```python
from build123d import *

# Parameters (mm, degrees)
SKETCH_W        = 70
SKETCH_H        = 70
PAD_DEPTH       = 15
SKETCH001_R     = 26
POCKET_DEPTH    = 11
SKETCH002_R     = 3
SKETCH002_R_2   = 21
POCKET001_DEPTH = 15.001


with BuildPart() as part:
    # Sketch → Pad (new body)
    with BuildSketch(Plane.XY):
        Rectangle(SKETCH_W, SKETCH_H)
    extrude(amount=PAD_DEPTH)

    # Sketch001 (on Face6 of Pad) → Pocket (cut)
    with BuildSketch(Plane.XY.offset(15)):
        Circle(SKETCH001_R)
    extrude(amount=-POCKET_DEPTH, mode=Mode.SUBTRACT)

    # Sketch002 → Pocket001 (cut, through all)
    with BuildSketch(Plane.XY.offset(15)):
        with Locations((-25, 25)):
            Circle(SKETCH002_R)
        with Locations((25, 25)):
            Circle(SKETCH002_R)
        with Locations((25, -25)):
            Circle(SKETCH002_R)
        with Locations((-25, -25)):
            Circle(SKETCH002_R)
        Circle(SKETCH002_R_2)
    extrude(amount=-POCKET001_DEPTH, mode=Mode.SUBTRACT)


solid = part.part
```
Check sheet for the modelled part. Datum: model origin and axes. Units: mm. A direction names the side the tool comes from. Round coordinates to 2 decimals unless told otherwise and drop trailing zeros. Write each loop counter-clockwise with the first axis right and the second up, starting at its lowest first coordinate (ties: lowest second). Pieces come first, ordered by that corner, then holes. Notation, with made-up numbers: M 78,84.25 L 129,84.25 A31 cw 129,109.25 Z; hole C 30.5,49 d9. An arc over 180 degrees is marked long. Write item = value, one per line. Start each with the question number.
1. Gauge pin test, flat ends, axial feed: pin 1 (25 mm diameter, centred on x = 0, y = 0, fed in from -Z); pin 2 (3 mm diameter, centred on x = 19.5, y = -19, fed in from -Z). Record the tip position at first contact, or that the pin passes through.
2. Scan lines: line 1 (Y direction, x = 0, z = 2.75); line 2 (Y direction, x = 8.5, z = 13.5); line 3 (Z direction, x = 6, y = 23). Record each from-to range of solid material in increasing order. Write a range as [from, to].
3. Section check D-D, the plane y = -25. Record the cut outline in (x, z), then the cut area to 3 significant figures.
4. Release check for a two-part mould opening along Y. For faces 1 (the flat face through (0, 35, 7)), 2 (the flat face through (15, -15, 0)), 3 (the cylindrical face through (-28, 25, 8)) record: pulls with the +Y half, pulls with the -Y half, needs draft (parallel to the pull), parting line crosses it, or undercut.
5. Section check B-B, the plane z = 2.75. Record the cut outline in (x, y).
6. Tool access check on faces 4 (the cylindrical face through (22, -25, 8)), 5 (the cylindrical face through (-20.633, -15.821, 9.577)). Record the directions out of +Z, -Z, +X, -X, +Y, -Y that give a thin tool (end or side, any length) a straight path to the whole face; none if there is none.
7. Section check A-A, the plane y = 0. Record the cut outline in (x, z).
Results found:
q1.pin_1 = through
q1.pin_2 = 0
q2.line_1 = [-35, -21], [21, 35]
q2.line_2 = [-35, -24.57], [24.57, 35]
q2.line_3 = [0, 4]
q3.outline = M -35,0 L -28,0 L -28,15 L -35,15 Z; M -22,0 L 22,0 L 22,15 L 7.14,15 L 7.14,4 L -7.14,4 L -7.14,15 L -22,15 Z; M 28,0 L 35,0 L 35,15 L 28,15 Z
q3.area = 713 mm^2
q4.face_1 = pulls with the +Y half
q4.face_2 = needs draft
q4.face_3 = undercut
q5.outline = M -35,-35 L 35,-35 L 35,35 L -35,35 Z; hole C -25,-25 d6; hole C -25,25 d6; hole C 0,0 d42; hole C 25,-25 d6; hole C 25,25 d6
q6.face_4 = +Z, -Z
q6.face_5 = +Z
q7.outline = M -35,0 L -21,0 L -21,4 L -26,4 L -26,15 L -35,15 Z; M 21,0 L 35,0 L 35,15 L 26,15 L 26,4 L 21,4 Z
